```python
from build123d import *

# Parameters (mm, degrees)
SKETCH2_R           = 1
BOSS_EXTRUDE1_DEPTH = 12


with BuildPart() as part:
    # Sketch2 → Boss-Extrude1 (new body)
    with BuildSketch(Plane.XY):
        Polygon((-0.25, 2.952368755), (0.25, 2.952368755), (0.375, 1.452368755), (0.550299562, 1.395410474), (1.533104565, 2.535462809), (1.937613062, 2.241570183), (1.157062308, 0.954571535), (1.265403395, 0.805452821), (2.730615294, 1.150096248), (2.885123791, 0.67456799), (1.497166141, 0.092160434), (1.497166141, -0.092160434), (2.885123791, -0.67456799), (2.730615294, -1.150096248), (1.265403395, -0.805452821), (1.157062308, -0.954571535), (1.937613062, -2.241570183), (1.533104565, -2.535462809), (0.550299562, -1.395410474), (0.375, -1.452368755), (0.25, -2.952368755), (-0.25, -2.952368755), (-0.375, -1.452368755), (-0.550299562, -1.395410474), (-1.533104565, -2.535462809), (-1.937613062, -2.241570183), (-1.157062308, -0.954571535), (-1.265403395, -0.805452821), (-2.730615294, -1.150096248), (-2.885123791, -0.67456799), (-1.497166141, -0.092160434), (-1.497166141, 0.092160434), (-2.885123791, 0.67456799), (-2.730615294, 1.150096248), (-1.265403395, 0.805452821), (-1.157062308, 0.954571535), (-1.937613062, 2.241570183), (-1.533104565, 2.535462809), (-0.550299562, 1.395410474), (-0.375, 1.452368755), align=None)
        Circle(SKETCH2_R, mode=Mode.SUBTRACT)
    extrude(amount=BOSS_EXTRUDE1_DEPTH)


solid = part.part
```
Source: CAD feature listing. Evaluate the final solid. Frame: model axes, mm. A direction names the side the tool comes from. Round coordinates to 2 decimals unless told otherwise and drop trailing zeros. Loops run counter-clockwise (first coordinate to the right, second up) from the corner with the lowest first, then second, coordinate; pieces in that order, holes last. Notation, with made-up numbers: M -28,15.5 L 0,15.5 A9 ccw 0,25.5 Z; hole C -13,-25.5 d9. An arc over 180 degrees is marked long. Use a Markdown table: item, result. Add a question column.
1. Mould query, pull axis Y, two halves, no side actions, for faces 1 (the flat face through (-0.313, 2.192, 5.916)), 2 (the flat face through (1.542, -1.589, 5.916)), 3 (the flat face through (-0.31, -2.21, 5.92)). Classes: pulls with the +Y half, pulls with the -Y half, needs draft (parallel to the pull), parting line crosses it, or undercut.
2. Reachability of faces 4 (the flat face through (1.049, -1.973, 5.916)), 5 (the flat face through (2.18, -0.38, 5.92)), 6 (the flat face through (2.01, -0.98, 5.92)), 7 (the flat face through (1.035, 1.957, 5.916)), 8 (the flat face through (-2.201, -0.387, 5.916)) from +Z, -Z, +X, -X, +Y, -Y: full face, straight path, thin tool, end or side. Return the list, or none.
3. Line query: line 1 (Y direction, x = 0, z = 5.25); line 2 (X direction, y = 1.55, z = 10); line 3 (Y direction, x = 1.8, z = 3.5). Output: solid intervals per line, ascending.
4. Section query B-B on x = -2.1. Return the cut outline in (y, z).
5. Contact query for a flat-ended pin moving along its axis: P1, Ø1, axis at y = -1.5, z = 5, coming from the +X side. Output: stop coordinate, or through.
6. Section query A-A on x = 0. Return the cut outline in (y, z).
Reported:
| question | item | result |
|---|---|---|
| 1 | face 1 | pulls with the +Y half |
| 1 | face 2 | undercut |
| 1 | face 3 | pulls with the -Y half |
| 2 | face 4 | +Z, -Z, -Y |
| 2 | face 5 | +Z, -Z, +X |
| 2 | face 6 | +Z, -Z |
| 2 | face 7 | +Z, -Z, +Y |
| 2 | face 8 | +Z, -Z, -X |
| 3 | line 1 | y = -2.95 to -1, 1 to 2.95 |
| 3 | line 2 | x = -1.52 to -0.68, -0.37 to 0.37, 0.68 to 1.52 |
| 3 | line 3 | y = -2.34 to -2.01, -0.93 to -0.22, 0.22 to 0.93, 2.01 to 2.34 |
| 4 | outline | M -1,0 L -0.35,0 L -0.35,12 L -1,12 Z; M 0.35,0 L 1,0 L 1,12 L 0.35,12 Z |
| 5 | P1 | stops at x = 2.78 |
| 6 | outline | M -2.95,0 L -1,0 L -1,12 L -2.95,12 Z; M 1,0 L 2.95,0 L 2.95,12 L 1,12 Z |
